from build123d import *

# Parameters (mm, degrees)
SKETCH_1_W          = 38
SKETCH_1_H          = 2.85
SKETCH_1_H_2        = 8.3
SKETCH_1_R          = 1.75
EXTRUDE_1_DEPTH     = 5
SKETCH_1_3_W        = 38
SKETCH_1_3_H        = 8.3
SKETCH_1_3_R        = 1.75
EXTRUDE_2_DEPTH     = 6.4
CUT_EXTRUDE_1_DEPTH = 2.5
FILLET_1_R          = 1
CHAMFER_1_SIZE      = 1.3
CHAMFER_1_SIZE_2    = 1.54927967


with BuildPart() as part:
    # Эскиз1 → Бобышка-Вытянуть1 (new body)
    # profile 1 of 3: a face of its own
    with BuildSketch(Plane.XY):
        with Locations((0, -5.575)):
            Rectangle(SKETCH_1_W, SKETCH_1_H)
    # profile 2 of 3: a face of its own
    with BuildSketch(Plane.XY):
        Rectangle(SKETCH_1_W, SKETCH_1_H_2)
        with Locations((-12.5, 0)):
            Circle(SKETCH_1_R, mode=Mode.SUBTRACT)
        with Locations((12.5, 0)):
            Circle(SKETCH_1_R, mode=Mode.SUBTRACT)
    # profile 3 of 3: a face of its own
    with BuildSketch(Plane.XY):
        with Locations((0, 5.575)):
            Rectangle(SKETCH_1_W, SKETCH_1_H)
    extrude(amount=EXTRUDE_1_DEPTH)

    # Эскиз1<3> → Бобышка-Вытянуть2 (add)
    with BuildSketch(Plane.XY):
        Rectangle(SKETCH_1_3_W, SKETCH_1_3_H)
        with Locations((-12.5, 0)):
            Circle(SKETCH_1_3_R, mode=Mode.SUBTRACT)
        with Locations((12.5, 0)):
            Circle(SKETCH_1_3_R, mode=Mode.SUBTRACT)
    extrude(amount=EXTRUDE_2_DEPTH)

    # Эскиз2 → Вырез-Вытянуть1 (cut)
    with BuildSketch(Plane(origin=(0, 0, 0), x_dir=(-1, 0, 0), z_dir=(0, 0, -1))):
        Polygon((-12.5, 3.348631561), (-15.4, 1.674315781), (-15.4, -1.674315781), (-12.5, -3.348631561), (-9.6, -1.674315781), (-9.6, 1.674315781), align=None)
        Polygon((9.6, 1.674315781), (12.5, 3.348631561), (15.4, 1.674315781), (15.4, -1.674315781), (12.5, -3.348631561), (9.6, -1.674315781), align=None)
    extrude(amount=-CUT_EXTRUDE_1_DEPTH, mode=Mode.SUBTRACT)

    # Скругление1
    fillet_1_edges = [part.edges().sort_by_distance(p)[0] for p in [
        (19, -7, 2.5),
        (-19, -7, 2.5),
        (-19, 7, 2.5),
        (19, 7, 2.5),
        (19, 4.15, 5.7),
        (-19, 4.15, 5.7),
        (-19, -4.15, 5.7),
        (19, -4.15, 5.7),
    ]]
    fillet(fillet_1_edges, radius=FILLET_1_R)

    # Фаска1
    # the kernel refuses this chamfer: 1.54927967, 1.3 mm, written as the material it takes off along each edge
    with BuildSketch(Plane(origin=(12.5, 0, 2.5), x_dir=(1, 0, 0), z_dir=(0, 1, 0))) as chamfer_1_piece_1_section:
        Polygon((1.75, -CHAMFER_1_SIZE), (1.75 + CHAMFER_1_SIZE_2, 0), (1.75, 0), align=None)
    chamfer_1_piece_1 = revolve(axis=Axis((12.5, 0, 2.5), (0, 0, -1)), mode=Mode.PRIVATE)
    chamfer_1_piece_1 = split(chamfer_1_piece_1, bisect_by=Plane(origin=(12.068379037, 3.597828041, 3.131156131), z_dir=(-0.4999999999999998, -0.8660254037844388, 0)), keep=Keep.TOP, mode=Mode.PRIVATE)
    chamfer_1_piece_1 = split(chamfer_1_piece_1, bisect_by=Plane(origin=(9.168379037, 1.425119301, 3.131156131), z_dir=(0.5000000000000004, -0.8660254037844385, 0)), keep=Keep.TOP, mode=Mode.PRIVATE)
    chamfer_1_piece_1 = split(chamfer_1_piece_1, bisect_by=Plane(origin=(15.4, 0, 3.131156131), z_dir=(-1, 0, 0)), keep=Keep.TOP, mode=Mode.PRIVATE)
    chamfer_1_piece_1 = split(chamfer_1_piece_1, bisect_by=Plane(origin=(9.6, 0, 3.131156131), z_dir=(1, 0, 0)), keep=Keep.TOP, mode=Mode.PRIVATE)
    chamfer_1_piece_1 = split(chamfer_1_piece_1, bisect_by=Plane(origin=(12.068379037, -3.597828041, 3.131156131), z_dir=(-0.4999999999999998, 0.8660254037844388, 0)), keep=Keep.TOP, mode=Mode.PRIVATE)
    chamfer_1_piece_1 = split(chamfer_1_piece_1, bisect_by=Plane(origin=(9.168379037, -1.425119301, 3.131156131), z_dir=(0.5000000000000001, 0.8660254037844386, 0)), keep=Keep.TOP, mode=Mode.PRIVATE)
    add(chamfer_1_piece_1, mode=Mode.SUBTRACT)
    with BuildSketch(Plane(origin=(-12.5, 0, 2.5), x_dir=(1, 0, 0), z_dir=(0, 1, 0))) as chamfer_1_piece_2_section:
        Polygon((1.75, -CHAMFER_1_SIZE), (1.75 + CHAMFER_1_SIZE_2, 0), (1.75, 0), align=None)
    chamfer_1_piece_2 = revolve(axis=Axis((-12.5, 0, 2.5), (0, 0, -1)), mode=Mode.PRIVATE)
    chamfer_1_piece_2 = split(chamfer_1_piece_2, bisect_by=Plane(origin=(-12.931620963, 3.597828041, 3.131156131), z_dir=(-0.5000000000000004, -0.8660254037844385, 0)), keep=Keep.TOP, mode=Mode.PRIVATE)
    chamfer_1_piece_2 = split(chamfer_1_piece_2, bisect_by=Plane(origin=(-9.6, 0, 3.131156131), z_dir=(-1, 0, 0)), keep=Keep.TOP, mode=Mode.PRIVATE)
    chamfer_1_piece_2 = split(chamfer_1_piece_2, bisect_by=Plane(origin=(-15.831620963, 1.425119301, 3.131156131), z_dir=(0.4999999999999998, -0.8660254037844388, 0)), keep=Keep.TOP, mode=Mode.PRIVATE)
    chamfer_1_piece_2 = split(chamfer_1_piece_2, bisect_by=Plane(origin=(-12.931620963, -3.597828041, 3.131156131), z_dir=(-0.5000000000000001, 0.8660254037844386, 0)), keep=Keep.TOP, mode=Mode.PRIVATE)
    chamfer_1_piece_2 = split(chamfer_1_piece_2, bisect_by=Plane(origin=(-15.4, 0, 3.131156131), z_dir=(1, 0, 0)), keep=Keep.TOP, mode=Mode.PRIVATE)
    chamfer_1_piece_2 = split(chamfer_1_piece_2, bisect_by=Plane(origin=(-15.831620963, -1.425119301, 3.131156131), z_dir=(0.4999999999999998, 0.8660254037844388, 0)), keep=Keep.TOP, mode=Mode.PRIVATE)
    add(chamfer_1_piece_2, mode=Mode.SUBTRACT)


solid = part.part
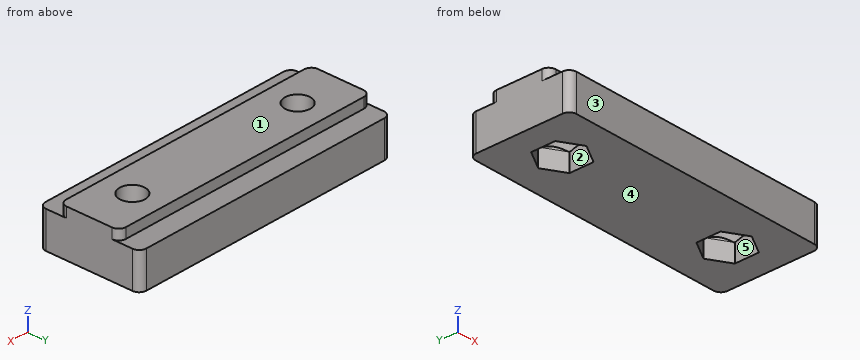
Input: part model. Units: mm. Frame: model coordinates. Face numbers are marked on the shaded views. A direction names the side the tool comes from. Coordinates: 2 decimals unless noted, no trailing zeros. Loops run counter-clockwise (first coordinate to the right, second up) from the corner with the lowest first, then second, coordinate; pieces in that order, holes last. Notation, with made-up numbers: (37.25, 42.25) -> (63.25, 42.25) arc R23 cw to (63.25, 81.25) -> close; hole circle Ø1 at (26.5, 71.25). An arc over 180 degrees is marked (long way). Write each question's results on one line, items separated by ' | '. Start each with the question number.
Q1. Section C-C, the plane y = 5.5. Return the cut outline in (x, z).
Q2. Section B-B, the plane x = 7.5. Return the cut outline in (y, z).
Q3. Ray query, line 1 (X direction, y = 0, z = 4.95); line 2 (Y direction, x = 12.5, z = 5.7); line 3 (X direction, y = -3, z = 1). Return the intervals inside material, ascending. Write a range as from..to.
Q4. Pull-direction query (Y, two-part tool) for the marked faces 1, 2 and 3; classes: released by +Y, released by -Y, zero draft, split by the parting line, or undercut.
Q5. Section A-A, the plane y = 0. Return the cut outline in (x, z), plus the area to 3 significant figures.
Q6. Reachability of the marked faces 4 and 5 from +Z, -Z, +X, -X, +Y, -Y: full face, straight path, thin tool, end or side. Return the list, or none.
Q7. Pin query (flat end, axial travel): pin 1 (1.9 mm diameter, centred on x = -6, y = 5, fed in from +Z); pin 2 (3 mm diameter, centred on x = 12.5, y = 0, fed in from +Z); pin 3 (0.7 mm diameter, centred on x = 2, z = 5.5, fed in from +Y). Return the tip coordinate at first contact, or that it passes through.
Found:
1) outline: (-19, 0) -> (19, 0) -> (19, 5) -> (-19, 5) -> close
2) outline: (-7, 0) -> (7, 0) -> (7, 5) -> (4.15, 5) -> (4.15, 6.4) -> (-4.15, 6.4) -> (-4.15, 5) -> (-7, 5) -> close
3) line 1: -19..-14.25, -10.75..10.75, 14.25..19 | line 2: -4.15..-1.75, 1.75..4.15 | line 3: -19..-13.1, -11.9..11.9, 13.1..19
4) face 1: zero draft | face 2: undercut | face 3: released by -Y
5) outline: (-19, 0) -> (-15.4, 0) -> (-15.4, 2.84) -> (-14.25, 3.8) -> (-14.25, 6.4) -> (-19, 6.4) -> close; (-10.75, 3.8) -> (-9.6, 2.84) -> (-9.6, 0) -> (9.6, 0) -> (9.6, 2.84) -> (10.75, 3.8) -> (10.75, 6.4) -> (-10.75, 6.4) -> close; (14.25, 3.8) -> (15.4, 2.84) -> (15.4, 0) -> (19, 0) -> (19, 6.4) -> (14.25, 6.4) -> close | area: 183 mm2
6) face 4: -Z, +X, -X, +Y, -Y | face 5: -Z
7) pin 1: z = 6.4 | pin 2: through | pin 3: y = 4.15
